```python
from build123d import *

# Parameters (mm, degrees)
SKETCH1_R           = 2.625
BOSS_EXTRUDE1_DEPTH = 5


with BuildPart() as part:
    # Sketch1 → Boss-Extrude1 (new body)
    with BuildSketch(Plane(origin=(0, 0, 0), x_dir=(1, 0, 0), z_dir=(0, 1, 0))):
        with BuildLine():
            Line((-42.535533906, 36.535533906), (-40.464466094, 34.464466094))
            ThreePointArc((-40.464466094, 34.464466094), (-39.380602337, 32.84234935), (-39, 30.928932188))
            Line((-39, 30.928932188), (-39, 19.071067812))
            ThreePointArc((-39, 19.071067812), (-39.380602337, 17.15765065), (-40.464466094, 15.535533906))
            Line((-40.464466094, 15.535533906), (-42.535533906, 13.464466094))
            ThreePointArc((-42.535533906, 13.464466094), (-43.619397663, 11.84234935), (-44, 9.928932188))
            Line((-44, 9.928932188), (-44, -9.928932188))
            ThreePointArc((-44, -9.928932188), (-43.619397663, -11.84234935), (-42.535533906, -13.464466094))
            Line((-42.535533906, -13.464466094), (-40.464466094, -15.535533906))
            ThreePointArc((-40.464466094, -15.535533906), (-39.380602337, -17.15765065), (-39, -19.071067812))
            Line((-39, -19.071067812), (-39, -30.928932188))
            ThreePointArc((-39, -30.928932188), (-39.380602337, -32.84234935), (-40.464466094, -34.464466094))
            Line((-40.464466094, -34.464466094), (-42.535533906, -36.535533906))
            ThreePointArc((-42.535533906, -36.535533906), (-43.619397663, -38.15765065), (-44, -40.071067812))
            Line((-44, -40.071067812), (-44, -45))
            ThreePointArc((-44, -45), (-42.535533906, -48.535533906), (-39, -50))
            Line((-39, -50), (-34.071067812, -50))
            ThreePointArc((-34.071067812, -50), (-32.15765065, -49.619397663), (-30.535533906, -48.535533906))
            Line((-30.535533906, -48.535533906), (-26.464466094, -44.464466094))
            ThreePointArc((-26.464466094, -44.464466094), (-24.84234935, -43.380602337), (-22.928932188, -43))
            Line((-22.928932188, -43), (22.928932188, -43))
            ThreePointArc((22.928932188, -43), (24.84234935, -43.380602337), (26.464466094, -44.464466094))
            Line((26.464466094, -44.464466094), (30.535533906, -48.535533906))
            ThreePointArc((30.535533906, -48.535533906), (32.15765065, -49.619397663), (34.071067812, -50))
            Line((34.071067812, -50), (39, -50))
            ThreePointArc((39, -50), (42.535533906, -48.535533906), (44, -45))
            Line((44, -45), (44, -40.071067812))
            ThreePointArc((44, -40.071067812), (43.619397663, -38.15765065), (42.535533906, -36.535533906))
            Line((42.535533906, -36.535533906), (40.464466094, -34.464466094))
            ThreePointArc((40.464466094, -34.464466094), (39.380602337, -32.84234935), (39, -30.928932188))
            Line((39, -30.928932188), (39, -19.071067812))
            ThreePointArc((39, -19.071067812), (39.380602337, -17.15765065), (40.464466094, -15.535533906))
            Line((40.464466094, -15.535533906), (42.535533906, -13.464466094))
            ThreePointArc((42.535533906, -13.464466094), (43.619397663, -11.84234935), (44, -9.928932188))
            Line((44, -9.928932188), (44, 9.928932188))
            ThreePointArc((44, 9.928932188), (43.619397663, 11.84234935), (42.535533906, 13.464466094))
            Line((42.535533906, 13.464466094), (40.464466094, 15.535533906))
            ThreePointArc((40.464466094, 15.535533906), (39.380602337, 17.15765065), (39, 19.071067812))
            Line((39, 19.071067812), (39, 30.928932188))
            ThreePointArc((39, 30.928932188), (39.380602337, 32.84234935), (40.464466094, 34.464466094))
            Line((40.464466094, 34.464466094), (42.535533906, 36.535533906))
            ThreePointArc((42.535533906, 36.535533906), (43.619397663, 38.15765065), (44, 40.071067812))
            Line((44, 40.071067812), (44, 45))
            ThreePointArc((44, 45), (42.535533906, 48.535533906), (39, 50))
            Line((39, 50), (34.071067812, 50))
            ThreePointArc((34.071067812, 50), (32.15765065, 49.619397663), (30.535533906, 48.535533906))
            Line((30.535533906, 48.535533906), (26.464466094, 44.464466094))
            ThreePointArc((26.464466094, 44.464466094), (24.84234935, 43.380602337), (22.928932188, 43))
            Line((22.928932188, 43), (21.931712199, 43))
            ThreePointArc((21.931712199, 43), (17.630549566, 45.450490243), (17.54536976, 50.4))
            ThreePointArc((17.54536976, 50.4), (19.795416719, 57.146672655), (19.542318227, 64.254150716))
            ThreePointArc((19.542318227, 64.254150716), (19.730044926, 66.105757405), (20.973665961, 67.490349535))
            Line((20.973665961, 67.490349535), (21.56863896, 67.833857356))
            ThreePointArc((21.56863896, 67.833857356), (22.966416439, 69.655476432), (22.666715171, 71.931933567))
            Line((22.666715171, 71.931933567), (21.666715171, 73.663984375))
            ThreePointArc((21.666715171, 73.663984375), (19.845096095, 75.061761854), (17.56863896, 74.762060586))
            Line((17.56863896, 74.762060586), (16.973665961, 74.418552765))
            ThreePointArc((16.973665961, 74.418552765), (15.152763485, 74.033841421), (13.455361705, 74.797068675))
            ThreePointArc((13.455361705, 74.797068675), (0, 80), (-13.455361705, 74.797068675))
            ThreePointArc((-13.455361705, 74.797068675), (-15.152763485, 74.033841421), (-16.973665961, 74.418552765))
            Line((-16.973665961, 74.418552765), (-17.56863896, 74.762060586))
            ThreePointArc((-17.56863896, 74.762060586), (-19.845096095, 75.061761854), (-21.666715171, 73.663984375))
            Line((-21.666715171, 73.663984375), (-22.666715171, 71.931933567))
            ThreePointArc((-22.666715171, 71.931933567), (-22.966416439, 69.655476432), (-21.56863896, 67.833857356))
            Line((-21.56863896, 67.833857356), (-20.973665961, 67.490349535))
            ThreePointArc((-20.973665961, 67.490349535), (-19.730044926, 66.105757405), (-19.542318227, 64.254150716))
            ThreePointArc((-19.542318227, 64.254150716), (-19.795416719, 57.146672655), (-17.54536976, 50.4))
            ThreePointArc((-17.54536976, 50.4), (-17.630549566, 45.450490243), (-21.931712199, 43))
            Line((-21.931712199, 43), (-22.928932188, 43))
            ThreePointArc((-22.928932188, 43), (-24.84234935, 43.380602337), (-26.464466094, 44.464466094))
            Line((-26.464466094, 44.464466094), (-30.535533906, 48.535533906))
            ThreePointArc((-30.535533906, 48.535533906), (-32.15765065, 49.619397663), (-34.071067812, 50))
            Line((-34.071067812, 50), (-39, 50))
            ThreePointArc((-39, 50), (-42.535533906, 48.535533906), (-44, 45))
            Line((-44, 45), (-44, 40.071067812))
            ThreePointArc((-44, 40.071067812), (-43.619397663, 38.15765065), (-42.535533906, 36.535533906))
        make_face()
        with Locations(Location((-39, 43, 0), (0, 0, 270))):
            Circle(SKETCH1_R, mode=Mode.SUBTRACT)
        with Locations(Location((-39, 7, 0), (0, 0, 270))):
            Circle(SKETCH1_R, mode=Mode.SUBTRACT)
        with Locations(Location((-39, -7, 0), (0, 0, 270))):
            Circle(SKETCH1_R, mode=Mode.SUBTRACT)
        with Locations(Location((-39, -43, 0), (0, 0, 270))):
            Circle(SKETCH1_R, mode=Mode.SUBTRACT)
        with Locations(Location((39, -43, 0), (0, 0, 270))):
            Circle(SKETCH1_R, mode=Mode.SUBTRACT)
        with Locations(Location((39, -7, 0), (0, 0, 270))):
            Circle(SKETCH1_R, mode=Mode.SUBTRACT)
        with Locations(Location((39, 7, 0), (0, 0, 270))):
            Circle(SKETCH1_R, mode=Mode.SUBTRACT)
        with Locations(Location((39, 43, 0), (0, 0, 270))):
            Circle(SKETCH1_R, mode=Mode.SUBTRACT)
        with Locations(Location((-5, 7, 0), (0, 0, 270))):
            Circle(SKETCH1_R, mode=Mode.SUBTRACT)
        with Locations(Location((5, 7, 0), (0, 0, 270))):
            Circle(SKETCH1_R, mode=Mode.SUBTRACT)
        with Locations(Location((5, -7, 0), (0, 0, 270))):
            Circle(SKETCH1_R, mode=Mode.SUBTRACT)
        with Locations(Location((-5, -7, 0), (0, 0, 270))):
            Circle(SKETCH1_R, mode=Mode.SUBTRACT)
    extrude(amount=BOSS_EXTRUDE1_DEPTH)


solid = part.part
```
Source: CAD feature listing. Evaluate the final solid. Frame: model axes, mm. A direction names the side the tool comes from. Give positions to 0.01 mm unless a question says otherwise; leave off trailing zeros. Loops run counter-clockwise (first coordinate to the right, second up) from the corner with the lowest first, then second, coordinate; pieces in that order, holes last. Notation, with made-up numbers: (18.25, -21) -> (66.25, -21) arc R22 cw to (66.25, -11) -> close; hole circle Ø8 at (5, -32). An arc over 180 degrees is marked (long way). Use a Markdown table: item, result. Add a question column.
(1) Section query A-A (z = 7). Output: boundary loops of the cut face in (x, y) (3 decimals), then the cut area to 3 significant figures.
(2) First-contact query: pin 1 Ø2.5 at (y, z) = (2.5, -23.5) entering from -X; pin 2 Ø2 at (x, y) = (-24.5, 3) entering from +Z; pin 3 Ø1.5 at (x, y) = (-22, 4) entering from -Z. Flat tips, straight axial feed; report the tip coordinate or a pass-through.
(3) Section query B-B (x = 5). Output: boundary loops of the cut face in (y, z) (3 decimals).
(4) Access query for faces 1 (the face through (17.668, 2.465, -45.388)), 2 (the face through (43.61, 2.46, -38.13)), 3 (the face through (28, 2, 46)), 4 (the face through (37, 2, -50)). Directions: +Z, -Z, +X, -X, +Y, -Y. A direction counts if a zero-diameter tool reaches every point of the face in a straight line with its end or side. Return the directions, or none.
(5) Ray query, line 1 (X direction, y = 1.65, z = 7) (3 decimals); line 2 (Z direction, x = 37, y = 3.1); line 3 (X direction, y = 3.6, z = -67.5). Return the intervals inside material, ascending.
(6) Section query C-C (y = 0.9). Count the separate pieces of the cut face and the enclosed holes in it, then the cut area to 3 significant figures.
(7) Pull-direction query (Z, two-part tool) for faces 5 (the face through (-43.61, 2.46, 38.13)), 6 (the face through (-44, 2, -43)), 7 (the face through (43, 2, -48)); classes: +Z half, -Z half, draft (parallel to the pull), parting line (faces both ways), or undercut.
Checked values:
| question | item | result |
|---|---|---|
| 1 | outline | (-44, 0) -> (-41.625, 0) -> (-41.625, 5) -> (-44, 5) -> close; (-36.375, 0) -> (-7.625, 0) -> (-7.625, 5) -> (-36.375, 5) -> close; (-2.375, 0) -> (2.375, 0) -> (2.375, 5) -> (-2.375, 5) -> close; (7.625, 0) -> (36.375, 0) -> (36.375, 5) -> (7.625, 5) -> close; (41.625, 0) -> (44, 0) -> (44, 5) -> (41.625, 5) -> close |
| 1 | area | 335 mm^2 |
| 2 | pin 1 | x = -39 |
| 2 | pin 2 | z = 43.71 |
| 2 | pin 3 | z = -74.22 |
| 3 | outline | (0, -79.365) -> (5, -79.365) -> (5, -9.625) -> (0, -9.625) -> close; (0, -4.375) -> (5, -4.375) -> (5, 4.375) -> (0, 4.375) -> close; (0, 9.625) -> (5, 9.625) -> (5, 43) -> (0, 43) -> close |
| 4 | face 1 | +Y, -Y |
| 4 | face 2 | +X, +Y, -Y |
| 4 | face 3 | +Z, +Y, -Y |
| 4 | face 4 | -Z, +X, +Y, -Y |
| 5 | line 1 | -44 to -41.625, -36.375 to -7.625, -2.375 to 2.375, 7.625 to 36.375, 41.625 to 44 |
| 5 | line 2 | -50 to -44.7, -41.3 to -8.7, -5.3 to 5.3, 8.7 to 41.3, 44.7 to 50 |
| 5 | line 3 | -20.99 to 20.99 |
| 6 | separate pieces | 1 |
| 6 | enclosed holes | 12 |
| 6 | area | 8,650 mm^2 |
| 7 | face 5 | undercut |
| 7 | face 6 | draft |
| 7 | face 7 | -Z half |
